Input: part model. Units: mm. Frame: model coordinates. Coordinates: 2 decimals unless noted, no trailing zeros. Loops run counter-clockwise (first coordinate to the right, second up) from the corner with the lowest first, then second, coordinate; pieces in that order, holes last. Notation, with made-up numbers: (42.25, 78.25) -> (87.25, 78.25) arc R27 cw to (87.25, 115.25) -> close; hole circle Ø1 at (81, -1.75). An arc over 180 degrees is marked (long way). Put each result on its own line as item: value. Start each with the question number.
1) Cut plane C-C (y = 13.5). Return the cut outline in (x, z).
2) Material intervals for L1, parallel to Y at x = 40, z = 3.5; L2, parallel to X at y = 186.5, z = 6, sorted ascending.
3) Contact query for flat-ended pins moving along their axis: P1, Ø6, axis at x = 186.5, y = 160, coming from the +Z side; P2, Ø4.5, axis at x = 40, y = 186.5, coming from the +Z side. Output: stop coordinate, or through.
4) Cut plane A-A (y = 160). Return the cut outline in (x, z).
from build123d import *

# Parameters (mm, degrees)
SKETCH_W   = 200
SKETCH_H   = 200
SKETCH_R   = 15
SKETCH_R_2 = 3
SKETCH_R_3 = 2.5
PAD_DEPTH  = 10
FILLET_R   = 3


with BuildPart() as part:
    # Sketch → Pad (new body)
    with BuildSketch(Plane.XY):
        with Locations((100, 100)):
            Rectangle(SKETCH_W, SKETCH_H)
        with Locations((136, 100)):
            Circle(SKETCH_R, mode=Mode.SUBTRACT)
        with Locations((118.32233, 117.67767)):
            Circle(SKETCH_R_2, mode=Mode.SUBTRACT)
        with Locations((153.67767, 117.67767)):
            Circle(SKETCH_R_2, mode=Mode.SUBTRACT)
        with Locations((118.32233, 82.32233)):
            Circle(SKETCH_R_2, mode=Mode.SUBTRACT)
        with Locations((153.67767, 82.32233)):
            Circle(SKETCH_R_2, mode=Mode.SUBTRACT)
        with Locations((40, 13.5)):
            Circle(SKETCH_R_3, mode=Mode.SUBTRACT)
        with Locations((160, 13.5)):
            Circle(SKETCH_R_3, mode=Mode.SUBTRACT)
        with Locations((80, 13.5)):
            Circle(SKETCH_R_3, mode=Mode.SUBTRACT)
        with Locations((120, 13.5)):
            Circle(SKETCH_R_3, mode=Mode.SUBTRACT)
        with Locations((40, 186.5)):
            Circle(SKETCH_R_3, mode=Mode.SUBTRACT)
        with Locations((80, 186.5)):
            Circle(SKETCH_R_3, mode=Mode.SUBTRACT)
        with Locations((120, 186.5)):
            Circle(SKETCH_R_3, mode=Mode.SUBTRACT)
        with Locations((160, 186.5)):
            Circle(SKETCH_R_3, mode=Mode.SUBTRACT)
        with Locations((13.5, 160)):
            Circle(SKETCH_R_3, mode=Mode.SUBTRACT)
        with Locations((13.5, 120)):
            Circle(SKETCH_R_3, mode=Mode.SUBTRACT)
        with Locations((13.5, 80)):
            Circle(SKETCH_R_3, mode=Mode.SUBTRACT)
        with Locations((13.5, 40)):
            Circle(SKETCH_R_3, mode=Mode.SUBTRACT)
        with Locations((186.5, 160)):
            Circle(SKETCH_R_3, mode=Mode.SUBTRACT)
        with Locations((186.5, 120)):
            Circle(SKETCH_R_3, mode=Mode.SUBTRACT)
        with Locations((186.5, 80)):
            Circle(SKETCH_R_3, mode=Mode.SUBTRACT)
        with Locations((186.5, 40)):
            Circle(SKETCH_R_3, mode=Mode.SUBTRACT)
    extrude(amount=PAD_DEPTH)

    # Fillet
    fillet_edges = [part.edges().sort_by_distance(p)[0] for p in [
        (0, 0, 5),
        (200, 0, 5),
        (0, 200, 5),
        (200, 200, 5),
    ]]
    fillet(fillet_edges, radius=FILLET_R)


solid = part.part
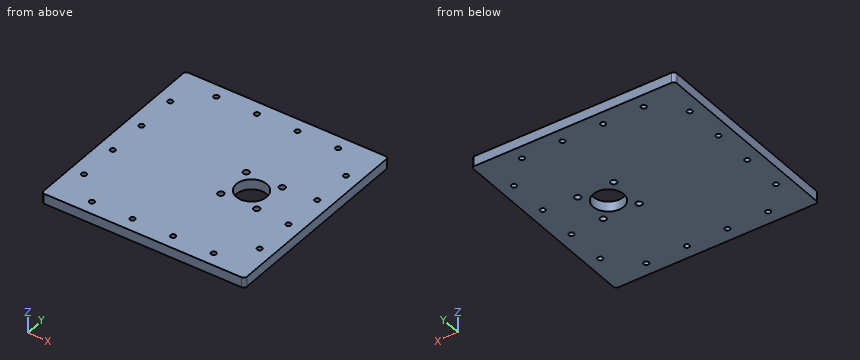
Results found:
1. outline: (0, 0) -> (37.5, 0) -> (37.5, 10) -> (0, 10) -> close; (42.5, 0) -> (77.5, 0) -> (77.5, 10) -> (42.5, 10) -> close; (82.5, 0) -> (117.5, 0) -> (117.5, 10) -> (82.5, 10) -> close; (122.5, 0) -> (157.5, 0) -> (157.5, 10) -> (122.5, 10) -> close; (162.5, 0) -> (200, 0) -> (200, 10) -> (162.5, 10) -> close
2. L1: y = 0 to 11, 16 to 184, 189 to 200
2. L2: x = 0 to 37.5, 42.5 to 77.5, 82.5 to 117.5, 122.5 to 157.5, 162.5 to 200
3. P1: stops at z = 10
3. P2: passes through
4. outline: (0, 0) -> (11, 0) -> (11, 10) -> (0, 10) -> close; (16, 0) -> (184, 0) -> (184, 10) -> (16, 10) -> close; (189, 0) -> (200, 0) -> (200, 10) -> (189, 10) -> close
